For this review, take the finished solid that the model builds, in its own axes (mm). Round coordinates to 2 decimals unless told otherwise and drop trailing zeros. Order: outer loops, then holes, each group sorted by start corner. A loop starts at its lowest first (then second) coordinate and runs counter-clockwise, first axis right, second up. Notation, with made-up numbers: M 62,-17 L 75,-17 A7 ccw 75,-11 Z; hole C 46.25,4.25 d9. An arc over 180 degrees is marked long. Answer as a JSON object with one key per item and string values.
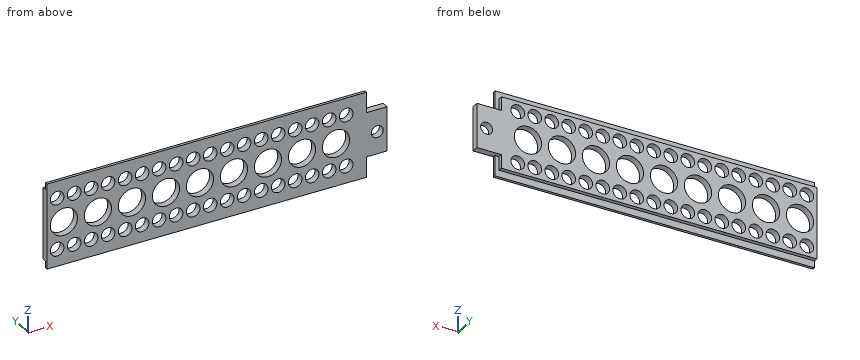
from build123d import *

# Parameters (mm, degrees)
SKIZZE1_W                       = 25
SKIZZE1_H                       = 2
AUFSATZ_LINEAR_AUSTRAGEN1_DEPTH = 100
SKIZZE2_W                       = 2
SKIZZE2_H                       = 1.2
SCHNITT_LINEAR_AUSTRAGEN1_DEPTH = 101
SKIZZE3_R                       = 1.75
SKIZZE3_W                       = 6
SKIZZE3_H                       = 6
SCHNITT_LINEAR_AUSTRAGEN2_DEPTH = 3
SKIZZE4_W                       = 4
SKIZZE4_H                       = 1.2
SCHNITT_LINEAR_AUSTRAGEN3_DEPTH = 1.2
SKIZZE5_R                       = 2
SKIZZE5_R_2                     = 4
SCHNITT_LINEAR_AUSTRAGEN4_DEPTH = 3
LINEARES_MUSTER1_COUNT          = 9
LINEARES_MUSTER1_PITCH          = 10


with BuildPart() as part:
    # Skizze1 → Aufsatz-Linear austragen1 (new body)
    with BuildSketch(Plane(origin=(0, 0, 0), x_dir=(0, 0, -1), z_dir=(1, 0, 0))):
        with Locations((-28.15591013, -26.369664989)):
            Rectangle(SKIZZE1_W, SKIZZE1_H)
    extrude(amount=AUFSATZ_LINEAR_AUSTRAGEN1_DEPTH)

    # Skizze2 → Schnitt-Linear austragen1 (cut, through all)
    with BuildSketch(Plane.ZY):
        with Locations((16.65591013, -25.969664989)):
            Rectangle(SKIZZE2_W, SKIZZE2_H)
        with Locations((39.65591013, -25.969664989)):
            Rectangle(SKIZZE2_W, SKIZZE2_H)
    extrude(amount=-SCHNITT_LINEAR_AUSTRAGEN1_DEPTH, mode=Mode.SUBTRACT)

    # Skizze3 → Schnitt-Linear austragen2 (cut, through all)
    with BuildSketch(Plane(origin=(0, -25.369664989, 0), x_dir=(1, 0, 0), z_dir=(0, 1, 0))):
        with Locations((97.15, -28.15591013)):
            Circle(SKIZZE3_R)
        with Locations((97, -18.65591013)):
            Rectangle(SKIZZE3_W, SKIZZE3_H)
        with Locations((97, -37.65591013)):
            Rectangle(SKIZZE3_W, SKIZZE3_H)
    extrude(amount=-SCHNITT_LINEAR_AUSTRAGEN2_DEPTH, mode=Mode.SUBTRACT)

    # Skizze4 → Schnitt-Linear austragen3 (cut)
    with BuildSketch(Plane(origin=(94, 0, 0), x_dir=(0, 0, -1), z_dir=(1, 0, 0))):
        with Locations((-36.65591013, -25.969664989)):
            Rectangle(SKIZZE4_W, SKIZZE4_H)
        with Locations((-19.65591013, -25.969664989)):
            Rectangle(SKIZZE4_W, SKIZZE4_H)
    extrude(amount=-SCHNITT_LINEAR_AUSTRAGEN3_DEPTH, mode=Mode.SUBTRACT)

    # Skizze5 → Schnitt-Linear austragen4 (cut, through all)
    with BuildSketch(Plane(origin=(0, -25.369664989, 0), x_dir=(1, 0, 0), z_dir=(0, 1, 0))):
        with Locations((3, -20.65591013)):
            Circle(SKIZZE5_R)
        with Locations((5, -28.15591013)):
            Circle(SKIZZE5_R_2)
        with Locations((3, -35.65591013)):
            Circle(SKIZZE5_R)
        with Locations((8, -35.65591013)):
            Circle(SKIZZE5_R)
        with Locations((8, -20.65591013)):
            Circle(SKIZZE5_R)
    schnitt_linear_austragen4 = extrude(amount=-SCHNITT_LINEAR_AUSTRAGEN4_DEPTH, mode=Mode.SUBTRACT)

    # Lineares Muster1: Schnitt-Linear austragen4 ×9
    with Locations(*[(i * LINEARES_MUSTER1_PITCH, 0, 0) for i in range(1, LINEARES_MUSTER1_COUNT)]):
        add(schnitt_linear_austragen4, mode=Mode.SUBTRACT)


solid = part.part
1) Add section A-A on x = 8. State the section outline as (y, z) points.
Geometry check:
{"outline": "M -27.37,15.66 L -26.57,15.66 L -26.57,17.66 L -25.37,17.66 L -25.37,18.66 L -27.37,18.66 Z; M -27.37,22.66 L -25.37,22.66 L -25.37,25.51 L -27.37,25.51 Z; M -27.37,30.8 L -25.37,30.8 L -25.37,33.66 L -27.37,33.66 Z; M -27.37,37.66 L -25.37,37.66 L -25.37,38.66 L -26.57,38.66 L -26.57,40.66 L -27.37,40.66 Z"}
2) Insertion check: P1, Ø3, axis at x = 18, z = 20.66, coming from the +Y side (1 decimal). The pin has a flat end and moves straight along its axis. Give the tip position at first contact, or say it passes through.
Geometry check:
{"P1": "passes through"}
3) For L1, parallel to Z at x = 43, y = -26.3; L2, parallel to Z at x = 78, y = -26.9; L3, parallel to Z at x = 95, y = -26.7, list the stretches that pass through material, from the lowest coordinate up.
Geometry check:
{"L1": "z = 17.66 to 18.66, 22.66 to 24.69, 31.62 to 33.66, 37.66 to 38.66", "L2": "z = 15.66 to 18.66, 22.66 to 25.51, 30.8 to 33.66, 37.66 to 40.66", "L3": "z = 21.66 to 34.66"}
4) Add section B-B on y = -25.7. State how many separate pieces and enclosed holes the cut face has, and give its area (3 significant figures).
Geometry check:
{"separate pieces": "1", "enclosed holes": "46", "area": "1,130 mm²"}
5) Add section C-C on x = 67.5. State the section outline as (y, z) points.
Geometry check:
{"outline": "M -27.37,15.66 L -26.57,15.66 L -26.57,17.66 L -25.37,17.66 L -25.37,18.72 L -27.37,18.72 Z; M -27.37,22.59 L -25.37,22.59 L -25.37,25.03 L -27.37,25.03 Z; M -27.37,31.28 L -25.37,31.28 L -25.37,33.72 L -27.37,33.72 Z; M -27.37,37.59 L -25.37,37.59 L -25.37,38.66 L -26.57,38.66 L -26.57,40.66 L -27.37,40.66 Z"}
